```python
from build123d import *

# Parameters (mm, degrees)
SKETCH12_W          = 50.8
SKETCH12_H          = 25.4
BOSS_EXTRUDE1_DEPTH = 7.62
SKETCH11_R          = 8.2696685
CUT_EXTRUDE2_DEPTH  = 8.62
SKETCH14_W          = 50.8
SKETCH14_H          = 19.05
BOSS_EXTRUDE2_DEPTH = 5.08


with BuildPart() as part:
    # Sketch12 → Boss-Extrude1 (new body)
    with BuildSketch(Plane.XY):
        with Locations((0, 12.7)):
            Rectangle(SKETCH12_W, SKETCH12_H)
    extrude(amount=BOSS_EXTRUDE1_DEPTH)

    # Sketch11 → Cut-Extrude2 (cut, through all)
    with BuildSketch(Plane.XY):
        with Locations((13.081, 12.7)):
            Circle(SKETCH11_R)
        with Locations((-13.081, 12.7)):
            Circle(SKETCH11_R)
    extrude(amount=CUT_EXTRUDE2_DEPTH, mode=Mode.SUBTRACT)

    # Sketch14 → Boss-Extrude2 (add)
    with BuildSketch(Plane(origin=(0, 0, 0), x_dir=(-1, 0, 0), z_dir=(0, -1, 0))):
        with Locations((0, 1.905)):
            Rectangle(SKETCH14_W, SKETCH14_H)
    extrude(amount=BOSS_EXTRUDE2_DEPTH)


solid = part.part
```
The model under review builds one solid part; all positions refer to its coordinate system, in mm. A direction names the side the tool comes from. Round coordinates to 2 decimals unless told otherwise and drop trailing zeros. Order: outer loops, then holes, each group sorted by start corner. A loop starts at its lowest first (then second) coordinate and runs counter-clockwise, first axis right, second up. Notation, with made-up numbers: (-19.75, 28) - (21.25, 28) arc R15 ccw to (21.25, 32) - close; hole circle Ø11 at (67, 49.5). An arc over 180 degrees is marked (long way). Answer in a Markdown table with one row per item.
(1) Machinability: for faces 5 (the face through (0, 13, 0)), 6 (the face through (0, -3, -11.43)), which of the approach directions +Z, -Z, +X, -X, +Y, -Y give a long, thin tool a straight path to every point of the face, cutting with its end or side? Answer none if there is none.
Result set:
| item | result |
|---|---|
| face 5 | -Z, +X, -X, +Y |
| face 6 | -Z, +X, -X, +Y, -Y |
(2) Take a section at D-D on x = -0.5. Write out the cut boundary in (y, z), plus the area to 3 significant figures.
Result set:
| item | result |
|---|---|
| outline | (-5.08, -11.43) - (0, -11.43) - (0, 0) - (25.4, 0) - (25.4, 7.62) - (-5.08, 7.62) - close |
| area | 290 mm2 |
(3) For line 1 (X direction, y = 12.7, z = 3.75); line 2 (Z direction, x = -8, y = 20); line 3 (X direction, y = 18, z = 0.25), list the stretches that pass through material, from the lowest coordinate up. Write a range as from..to.
Result set:
| item | result |
|---|---|
| line 1 | x = -25.4..-21.35, -4.81..4.81, 21.35..25.4 |
| line 2 | z = 0..7.62 |
| line 3 | x = -25.4..-19.43, -6.73..6.73, 19.43..25.4 |
(4) Take a section at B-B on z = 6. Write out the cut boundary in (x, y), plus the area to 3 significant figures.
Result set:
| item | result |
|---|---|
| outline | (-25.4, -5.08) - (25.4, -5.08) - (25.4, 25.4) - (-25.4, 25.4) - close; hole circle Ø16.54 at (-13.08, 12.7); hole circle Ø16.54 at (13.08, 12.7) |
| area | 1,120 mm2 |
(5) Mouldability with a two-part tool opening along X and no side actions: class faces 1 (the face through (16.897, 5.363, 3.757)), 2 (the face through (-14.874, 4.627, 3.757)), 3 (the face through (0, -5.08, -2)), 4 (the face through (-25.4, 10, 2)) as released by +X, released by -X, zero draft, split by the parting line, or undercut.
Result set:
| item | result |
|---|---|
| face 1 | undercut |
| face 2 | undercut |
| face 3 | zero draft |
| face 4 | released by -X |
(6) Take a section at A-A on y = 12.7. Write out the cut boundary in (x, z).
Result set:
| item | result |
|---|---|
| outline | (-25.4, 0) - (-21.35, 0) - (-21.35, 7.62) - (-25.4, 7.62) - close; (-4.81, 0) - (4.81, 0) - (4.81, 7.62) - (-4.81, 7.62) - close; (21.35, 0) - (25.4, 0) - (25.4, 7.62) - (21.35, 7.62) - close |
(7) Clearance check with flat-ended pins moving along their axes: P1, Ø5, axis at x = 8.5, y = 12, coming from the -Z side; P2, Ø5, axis at x = 15.5, z = -7, coming from the +Y side; P3, Ø12.5, axis at x = -11.5, y = 16, coming from the -Z side. State where each tip first meets the part, or that it passes through.
Result set:
| item | result |
|---|---|
| P1 | passes through |
| P2 | stops at y = 0 |
| P3 | stops at z = 0 |
(8) Take a section at C-C on x = -15.5. Write out the cut boundary in (y, z), plus the area to 3 significant figures.
Result set:
| item | result |
|---|---|
| outline | (-5.08, -11.43) - (0, -11.43) - (0, 0) - (4.79, 0) - (4.79, 7.62) - (-5.08, 7.62) - close; (20.61, 0) - (25.4, 0) - (25.4, 7.62) - (20.61, 7.62) - close |
| area | 170 mm2 |
